```python
from build123d import *

# Parameters (mm, degrees)
F0_W     = 400
F0_H     = 352
F1_DEPTH = 19
F3_DEPTH = 19.001
F5_DEPTH = 19.0010001
F6_W     = 14.9907767773
F6_H     = 28.43076922
F7_DEPTH = 19.0010001


with BuildPart() as f1:
    # F0 (on Top) → F1 (new body)
    with BuildSketch(Plane.XY):
        Rectangle(F0_W, F0_H)
    extrude(amount=F1_DEPTH)

    # F2 (on face) → F3 (cut, through all)
    with BuildSketch(Plane.XY.offset(19)):
        with BuildLine():
            add(Edge.make_bspline(
                [(-200, -23.7784627825), (-126.5126396068, -24.453447739), (6.9760460018, -25.6795477673), (2.163274492, -129.3855711593), (0, -176)],
                knots=[0, 0, 0, 0, 0.5505137762, 1, 1, 1, 1], degree=3))
            Line((-200, -23.7784627825), (-200, -176))
            Line((-200, -176), (0, -176))
        make_face()
        with BuildLine():
            Line((-200, 176), (-200, 25.8461534977))
            add(Edge.make_bspline(
                [(-200, 25.8461534977), (-125.0792777845, 25.7364442733), (10.3974148662, 25.5380606696), (3.211839993, 129.5211703688), (0, 176)],
                knots=[0, 0, 0, 0, 0.5530155833, 1, 1, 1, 1], degree=3))
            Line((0, 176), (-200, 176))
        make_face()
    extrude(amount=-F3_DEPTH, mode=Mode.SUBTRACT)

    # F4 (on face) → F5 (cut, through all)
    with BuildSketch(Plane.XY.offset(19)):
        with BuildLine():
            ThreePointArc((177.3485280662, 176), (193.531261968, 165.4340185307), (200, 147.2220370564))
            Line((200, 147.2220370564), (200, 176))
            Line((200, 176), (177.3485280662, 176))
        make_face()
        with BuildLine():
            ThreePointArc((200, -143.14840734), (182.1787262713, -163.5266665451), (158.1519246101, -176))
            Line((158.1519246101, -176), (200, -176))
            Line((200, -176), (200, -143.14840734))
        make_face()
    extrude(amount=-F5_DEPTH, mode=Mode.SUBTRACT)

    # F6 (on face) → F7 (cut, through all)
    with BuildSketch(Plane.XY.offset(19)):
        with Locations((-176.2707680464, 1.8092310056)):
            Rectangle(F6_W, F6_H)
    extrude(amount=-F7_DEPTH, mode=Mode.SUBTRACT)


solid = f1.part
```
CAD build for the part. Positions are in the model's coordinates, mm. A direction names the side the tool comes from. Round coordinates to 2 decimals unless told otherwise and drop trailing zeros. Order: outer loops, then holes, each group sorted by start corner. A loop starts at its lowest first (then second) coordinate and runs counter-clockwise, first axis right, second up.
Q1. Slice it at A-A (y = 3.5). Write the cut outline in (x, z), and give its area (3 significant figures).
Q2. Two-plate mould, pull along X, no slides. Class faces 1 (the flat face through (-200, 1, 9)), 2 (the flat face through (-183.766, 2, 10)), 3 (the cylindrical face through (182.48, -163.29, 9.63)), 4 (the flat face through (86, 2, 0)): pulls with the +X half, pulls with the -X half, needs draft (parallel to the pull), parting line crosses it, or undercut.
Q3. Drop flat-ended pins along their axis: pin 1 (1 mm diameter, centred on x = -95, z = 3.5, fed in from +Y); pin 2 (4.5 mm diameter, centred on x = -174.5, z = 11.5, fed in from +Y). Give the stop position or say it passes through.
Q4. Which spindle directions (+Z, -Z, +X, -X, +Y, -Y) get a long thin tool onto all of the face, cutting with end or side? Do faces 5 (the flat face through (-168.775, 2, 10)), 6 (the flat face through (78, -176, 9)). Say none if no direction does.
Q5. Wall check: L1, parallel to X at y = -5, z = 17; L2, parallel to X at y = -134.5, z = 2.75; L3, parallel to Y at x = -27, z = 2. Give the ranges that are in metal, low to high.
Results below:
1. outline: (-200, 0) - (-183.77, 0) - (-183.77, 19) - (-200, 19) - close; (-168.78, 0) - (200, 0) - (200, 19) - (-168.78, 19) - close
1. area: 7,320 mm2
2. face 1: pulls with the -X half
2. face 2: undercut
2. face 3: pulls with the +X half
2. face 4: needs draft
3. pin 1: stops at y = 29.49
3. pin 2: stops at y = 25.87
4. face 5: +Z, -Z
4. face 6: +Z, -Z, +X, -X, -Y
5. L1: x = -200 to -183.77, -168.78 to 200
5. L2: x = 1.19 to 200
5. L3: y = -51.93 to 50.49
